Design review of the part built by this model. Coordinates are the model's own, in mm. Round coordinates to 2 decimals unless told otherwise and drop trailing zeros. Loops run counter-clockwise (first coordinate to the right, second up) from the corner with the lowest first, then second, coordinate; pieces in that order, holes last. Notation, with made-up numbers: (62, -11.75) -> (82, -11.75) arc R14 cw to (82, 12.25) -> close; hole circle Ø3 at (-28, 71). An arc over 180 degrees is marked (long way). Write each question's results on one line, items separated by ' | '. Start each with the question number.
from build123d import *

# Parameters (mm, degrees)
SKETCH002_R         = 1.75
POCKET_DEPTH        = 25.000541
POCKET_DEPTH_BACK   = 1.000982
LINEARPATTERN_COUNT = 2
LINEARPATTERN_PITCH = 125


with BuildPart() as part:
    # Sketch → AdditiveLoft section 0
    with BuildSketch(Plane.XZ):
        Polygon((0, 0), (24, 0), (24, 15), (22.4, 15), (22.4, 0.8), (1.6, 0.8), (1.6, 7.5), (0, 7.5), align=None)
    # Sketch001 (on DatumPlane) → AdditiveLoft section 1
    with BuildSketch(Plane.XZ.offset(165)):
        Polygon((0, 0), (0, 7.5), (1.6, 7.5), (1.6, 0.8), (23.4, 0.8), (23.4, 15), (25, 15), (25, 0), align=None)
    loft()

    # Sketch002 (on Face4 of AdditiveLoft) → Pocket (cut, two sides)
    with BuildSketch(Plane(origin=(23.999118, 0.145449, 0), x_dir=(0, 0, 1), z_dir=(0.999982, 0.00606, 0))) as pocket_sk:
        with Locations((3.5, 20)):
            Circle(SKETCH002_R)
    pocket = extrude(amount=-POCKET_DEPTH, mode=Mode.SUBTRACT) + extrude(pocket_sk.sketch, amount=POCKET_DEPTH_BACK, mode=Mode.SUBTRACT)

    # LinearPattern: Pocket ×2
    with Locations(*[(0, -i * LINEARPATTERN_PITCH, 0) for i in range(1, LINEARPATTERN_COUNT)]):
        add(pocket, mode=Mode.SUBTRACT)


solid = part.part
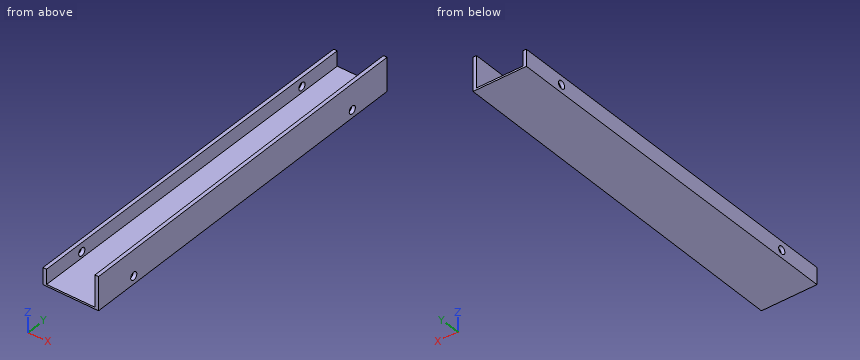
1) To check wall thickness, follow line 1 (X direction, y = -17.5, z = 2.5); line 2 (Z direction, x = 22.75, y = -65); line 3 (X direction, y = -145, z = 9.5). State the ranges of each line that lie inside material, in increasing order. Write a range as from..to.
2) Insertion check: pin 1 (1.3 mm diameter, centred on x = 0.5, y = -43.5, fed in from +Z); pin 2 (5 mm diameter, centred on y = -102.5, z = 8.5, fed in from +X); pin 3 (3.5 mm diameter, centred on y = -60, z = 2.5, fed in from +X); pin 4 (3 mm diameter, centred on x = 6, z = 4, fed in from -Y). Each pin has a flat end and moves straight along its axis. Give the tip position at first contact, or say it passes through.
3) Take a section at A-A (z = 3.5). Write out the cut boundary in (x, y), plus the area to 3 significant figures.
4) Take a section at B-B (z = 13.25). Write out the cut boundary in (x, y), plus the area to 3 significant figures.
Geometry check:
1) line 1: x = 0..1.6, 22.51..24.11 | line 2: z = 0..0.8 | line 3: x = 23.28..24.88
2) pin 1: stops at z = 7.5 | pin 2: stops at x = 24.64 | pin 3: stops at x = 24.37 | pin 4: passes through
3) outline: (0, -165) -> (1.6, -165) -> (1.6, -146.74) -> (0, -146.75) -> close; (0, -143.25) -> (1.6, -143.24) -> (1.6, -21.74) -> (0, -21.75) -> close; (0, -18.25) -> (1.6, -18.24) -> (1.6, 0) -> (0, 0) -> close; (22.4, 0) -> (22.51, -18.11) -> (24.11, -18.1) -> (24, 0) -> close; (22.53, -21.61) -> (23.27, -143.11) -> (24.87, -143.1) -> (24.13, -21.6) -> close; (23.29, -146.61) -> (23.4, -165) -> (25, -165) -> (24.89, -146.6) -> close | area: 506 mm^2
4) outline: (22.4, 0) -> (23.4, -165) -> (25, -165) -> (24, 0) -> close | area: 264 mm^2
